```python
from build123d import *

# Parameters (mm, degrees)
F0_R     = 14
F0_W     = 9.5
F0_H     = 9.5
F1_DEPTH = 3.4
F0_R_2   = 3.7
F2_DEPTH = 4.6


# Not quite as in the source:
# - a fillet or chamfer that OpenCascade refuses, or shapes differently, is made with other operations: its cross-section is extruded or revolved along the edge and cut away or added


with BuildPart() as f1:
    # F0 (on Top) → F1 (new body)
    with BuildSketch(Plane.XY):
        Circle(F0_R)
        Rectangle(F0_W, F0_H, mode=Mode.SUBTRACT)
    extrude(amount=F1_DEPTH)

    # F0 (on Top) → F2 (join)
    with BuildSketch(Plane.XY):
        Rectangle(F0_W, F0_H)
        Circle(F0_R_2, mode=Mode.SUBTRACT)
    extrude(amount=F2_DEPTH)

    # F3: chamfer of 5.5 x 4.6150479715 on 1 edges, made by hand

    # F3_s1 → F3_t2 (revolve, cut)
    with BuildSketch(Plane.XZ):
        Polygon((14, -1.2150479715), (8.5, 3.4), (14, 3.4), align=None)
    revolve(axis=Axis((0, 0, 3.4), (0, 0, 1)), mode=Mode.SUBTRACT)


solid = f1.part
```
Part model, mm, in its own coordinate system. A direction names the side the tool comes from. Give positions to 0.01 mm unless a question says otherwise; leave off trailing zeros. Loops run counter-clockwise (first coordinate to the right, second up) from the corner with the lowest first, then second, coordinate; pieces in that order, holes last. Notation, with made-up numbers: M -33,44.25 L -18,44.25 A14 cw -18,55.25 Z; hole C 12.25,-1.5 d11. An arc over 180 degrees is marked long. Return JSON: item names as keys, results as strings.
1) Pull direction X, two halves, no side cores. Call faces 1 (the face through (-2.2, 3.2, 4.6)), 2 (the face through (-4.75, 0, 4)), 3 (the face through (-0.802, -3.612, 2.268)), 4 (the face through (-6.901, -5.292, 3.235)): released by +X, released by -X, zero draft, split by the parting line, or undercut.
Calculated:
{"face 1": "zero draft", "face 2": "released by -X", "face 3": "undercut", "face 4": "split by the parting line"}
2) Saw through at A-A, the plane y = 0. List the corners of the cut face in (x, z).
Calculated:
{"outline": "M -12.55,0 L -3.7,0 L -3.7,4.6 L -4.75,4.6 L -4.75,3.4 L -8.5,3.4 Z; M 3.7,0 L 12.55,0 L 8.5,3.4 L 4.75,3.4 L 4.75,4.6 L 3.7,4.6 Z"}
3) Saw through at D-D, the plane z = 0.55. List the corners of the cut face in (x, y), then the cut area to 3 significant figures.
Calculated:
{"outline": "C 0,0 d23.79; hole C 0,0 d7.4", "area": "402 mm2"}
4) 3-axis set-ups, long thin cutter, end or side, ignore diameter. For faces 5 (the face through (0, -4.75, 4)), 6 (the face through (3, 3, 0)), 7 (the face through (0, 4.75, 4)), 8 (the face through (4.75, 0, 4)): which of +Z, -Z, +X, -X, +Y, -Y reach the whole face in a straight line?
Calculated:
{"face 5": "+Z, +X, -X, -Y", "face 6": "-Z, +X, -X, +Y, -Y", "face 7": "+Z, +X, -X, +Y", "face 8": "+Z, +X, +Y, -Y"}
5) Saw through at C-C, the plane z = 2.3. List the corners of the cut face in (x, y).
Calculated:
{"outline": "C 0,0 d19.62; hole C 0,0 d7.4"}
6) Flat gauge pins, fed straight in: pin 1 Ø8 at (x, y) = (9.5, 7) entering from +Z; pin 2 Ø1 at (x, y) = (-6.5, 7.5) entering from +Z; pin 3 Ø1.5 at (x, y) = (-3.5, -6.5) entering from -Z; pin 4 Ø0.6 at (y, z) = (1, 4) entering from -X. Where does each tip first touch, or does it go through?
Calculated:
{"pin 1": "stops at z = 3.4", "pin 2": "stops at z = 2.62", "pin 3": "stops at z = 0", "pin 4": "stops at x = -4.75"}
7) Drill centre lines: line 1 (Z direction, x = 5.25, y = -4.5); line 2 (Y direction, x = -1, z = 3.2); line 3 (X direction, y = 3, z = 2.1). Where is each one in solid material? Low to high.
Calculated:
{"line 1": "z = 0 to 3.4", "line 2": "y = -8.68 to -3.56, 3.56 to 8.68", "line 3": "x = -9.59 to -2.17, 2.17 to 9.59"}
